Part model, mm, in its own coordinate system. A direction names the side the tool comes from. Give positions to 0.01 mm unless a question says otherwise; leave off trailing zeros. Write each loop counter-clockwise with the first axis right and the second up, starting at its lowest first coordinate (ties: lowest second). Pieces come first, ordered by that corner, then holes.
```python
from build123d import *

# Parameters (mm, degrees)
SKETCH1_W           = 416.08
SKETCH1_H           = 314.48
BOSS_EXTRUDE2_DEPTH = 101.6
SKETCH2_W           = 403.38
SKETCH2_H           = 308.13
CUT_EXTRUDE1_DEPTH  = 320.090106675
CUT_EXTRUDE2_DEPTH  = 462.687674829
CUT_EXTRUDE3_REACH  = 415.528
SKETCH4_W           = 111.28
SKETCH4_H           = 38.1
SKETCH5_W           = 403.38
SKETCH5_H           = 12.7
BOSS_EXTRUDE3_DEPTH = 308.13


with BuildPart() as part:
    # Sketch1 → Boss-Extrude2 (new body)
    with BuildSketch(Plane(origin=(0, 0, 0), x_dir=(1, 0, 0), z_dir=(0, 1, 0))):
        with Locations((40.527, 15.127)):
            Rectangle(SKETCH1_W, SKETCH1_H)
    extrude(amount=BOSS_EXTRUDE2_DEPTH)

    # Sketch2 → Cut-Extrude1 (cut, through all)
    with BuildSketch(Plane(origin=(0, 101.6, 0), x_dir=(1, 0, 0), z_dir=(0, 1, 0))):
        with Locations((40.527, 18.302)):
            Rectangle(SKETCH2_W, SKETCH2_H)
    extrude(amount=-CUT_EXTRUDE1_DEPTH, mode=Mode.SUBTRACT)

    # Sketch3 → Cut-Extrude2 (cut, through all)
    with BuildSketch(Plane(origin=(248.567, 0, 0), x_dir=(0, 0, -1), z_dir=(1, 0, 0))):
        with BuildLine():
            Line((-142.113, 63.5), (-142.113, 101.6))
            Line((-142.113, 101.6), (172.367, 101.6))
            Line((172.367, 101.6), (-65.913, 88.9))
            ThreePointArc((-65.913, 88.9), (-105.728307199, 81.345921598), (-142.113, 63.5))
        make_face()
    extrude(amount=-CUT_EXTRUDE2_DEPTH, mode=Mode.SUBTRACT)

    # Sketch4 → Cut-Extrude3 (cut, up to next)
    with BuildSketch(Plane.XY.offset(142.113), mode=Mode.PRIVATE) as cut_extrude3_sk1:
        with Locations((40.527, 19.05)):
            Rectangle(SKETCH4_W, SKETCH4_H)
    cut_extrude3_tool1 = extrude(cut_extrude3_sk1.sketch, amount=-CUT_EXTRUDE3_REACH, mode=Mode.PRIVATE) & part.part
    add(cut_extrude3_tool1.solids().sort_by_distance((40.527, 19.05, 142.113))[0], mode=Mode.SUBTRACT)

    # Sketch5 → Boss-Extrude3 (add)
    with BuildSketch(Plane(origin=(0, 0, 135.763), x_dir=(-1, 0, 0), z_dir=(0, 0, -1))):
        with Locations((-40.527, 44.45)):
            Rectangle(SKETCH5_W, SKETCH5_H)
    extrude(amount=BOSS_EXTRUDE3_DEPTH)


solid = part.part
```
1) Saw through at B-B, the plane x = 173. Write the cut outline in (y, z), then the cut area to 3 significant figures.
Answers follow:
outline: (0, 135.76) - (38.1, 135.76) - (38.1, -172.37) - (50.8, -172.37) - (50.8, 135.76) - (67.53, 135.76) arc R151.39 ccw to (63.5, 142.11) - (0, 142.11) - close
area: 4,330 mm2
2) Saw through at D-D, the plane z = 45. Write the cut outline in (x, y).
Answers follow:
outline: (-167.51, 0) - (-161.16, 0) - (-161.16, 38.1) - (242.22, 38.1) - (242.22, 0) - (248.57, 0) - (248.57, 90.01) - (242.22, 90.01) - (242.22, 50.8) - (-161.16, 50.8) - (-161.16, 90.01) - (-167.51, 90.01) - close
3) Saw through at C-C, the plane y = 58. Write the cut outline in (x, z), then the cut area to 3 significant figures.
Answers follow:
outline: (-167.51, -172.37) - (-161.16, -172.37) - (-161.16, 135.76) - (242.22, 135.76) - (242.22, -172.37) - (248.57, -172.37) - (248.57, 142.11) - (-167.51, 142.11) - close
area: 6,560 mm2
4) Saw through at A-A, the plane y = 31. Write the cut outline in (x, z), then the cut area to 3 significant figures.
Answers follow:
outline: (-167.51, -172.37) - (-161.16, -172.37) - (-161.16, 135.76) - (-15.11, 135.76) - (-15.11, 142.11) - (-167.51, 142.11) - close; (96.17, 135.76) - (242.22, 135.76) - (242.22, -172.37) - (248.57, -172.37) - (248.57, 142.11) - (96.17, 142.11) - close
area: 5,850 mm2
5) Two-plate mould, pull along X, no slides. Class faces 1 (the face through (41, 44, -172.367)), 2 (the face through (248.567, 50, -13)), 3 (the face through (168, 19, 135.763)): +X half, -X half, draft (parallel to the pull), parting line (faces both ways), or undercut.
Answers follow:
face 1: draft
face 2: +X half
face 3: undercut
6) Pin check, flat tips, straight feed: pin 1 Ø8 at (x, y) = (-41, 15.5) entering from -Z; pin 2 Ø4 at (x, z) = (140, 28) entering from -Y. Stop position of each tip, or through.
Answers follow:
pin 1: stops at z = 135.76
pin 2: stops at y = 38.1
7) Wall check: L1, parallel to X at y = 26, z = -117.5; L2, parallel to Z at x = 106.5, y = 62; L3, parallel to Y at x = 125.5, z = -73. Give the ranges that are in metal, low to high.
Answers follow:
L1: x = -167.51 to -161.16, 242.22 to 248.57
L2: z = 135.76 to 142.11
L3: y = 38.1 to 50.8
8) 3-axis set-ups, long thin cutter, end or side, ignore diameter. For faces 4 (the face through (43, 50.8, -16)), 5 (the face through (-161.163, 19, -16)), 6 (the face through (41.5, 66.06, 138.16)): which of +Z, -Z, +X, -X, +Y, -Y reach the whole face in a straight line?
Answers follow:
face 4: -Z, +Y
face 5: -Z, -Y
face 6: +Z, +X, -X, +Y
